Geometry check sheet. Reference: the model listing, model coordinates, mm. A direction names the side the tool comes from. Round coordinates to 2 decimals unless told otherwise and drop trailing zeros. Loops run counter-clockwise (first coordinate to the right, second up) from the corner with the lowest first, then second, coordinate; pieces in that order, holes last.
```python
from build123d import *

# Parameters (mm, degrees)
BOSS_EXTRUDE1_DEPTH      = 125
BOSS_EXTRUDE1_DEPTH_BACK = 75
SKETCH1_R                = 10
BOSS_EXTRUDE2_START      = 15
BOSS_EXTRUDE2_DEPTH      = 7.5
BODY_MOVE_COPY4_ANGLE    = 90
CUT_EXTRUDE1_START       = 10
CUT_EXTRUDE1_DEPTH       = 4
CUT_EXTRUDE1_DRAFT       = -5


with BuildPart() as part:
    # Sketch1 → Boss-Extrude1 (new, two sides: drawn at the far end of the back side and taken through both)
    with BuildSketch(Plane(origin=(0, 0, 0), x_dir=(0, 0, -1), z_dir=(1, 0, 0)).offset(-BOSS_EXTRUDE1_DEPTH_BACK)):
        Circle(SKETCH1_R)
    extrude(amount=BOSS_EXTRUDE1_DEPTH + BOSS_EXTRUDE1_DEPTH_BACK)

    # Sketch2 → Boss-Extrude2 (add, symmetric)
    with BuildSketch(Plane(origin=(0, 0, 0), x_dir=(0, 0, -1), z_dir=(1, 0, 0)).offset(BOSS_EXTRUDE2_START)):
        with BuildLine():
            ThreePointArc((-4.950818385, 10.931120589), (-10.855235073, -5.115063196), (5.27814522, -10.776881879))
            ThreePointArc((5.27814522, -10.776881879), (10.675009162, -7.586625818), (15.507108825, -3.59229396))
            ThreePointArc((15.507108825, -3.59229396), (16.895326586, -1.149524968), (16.746983201, 1.656230392))
            ThreePointArc((16.746983201, 1.656230392), (7.939134659, 11.068540296), (-4.950818385, 10.931120589))
        make_face()
    boss_extrude2 = extrude(amount=BOSS_EXTRUDE2_DEPTH, both=True)

    # Mirror3: Boss-Extrude2 across plane
    add(boss_extrude2.mirror(Plane(origin=(0, 0, 0), x_dir=(0, 0, 1), z_dir=(1, 0, 0))))


with BuildPart() as body_2:
    # Split1: the piece on the far side of the plane
    add(part.part)
    split(bisect_by=Plane(origin=(0, 0, 0), x_dir=(0, 0, 1), z_dir=(1, 0, 0)), keep=Keep.BOTTOM)


with BuildPart() as part_1:
    add(part.part)

    # Split1
    split(bisect_by=Plane(origin=(0, 0, 0), x_dir=(0, 0, 1), z_dir=(1, 0, 0)), keep=Keep.TOP)


with BuildPart() as body_2_1:
    # Body-Move/Copy4: moved
    add(body_2.part.rotate(Axis((0, 0, 0), (-1, 0, 0)), BODY_MOVE_COPY4_ANGLE))

    # Combine1: union part
    add(part_1.part)


with BuildPart() as cut_extrude1_tool:
    # Sketch5 → Cut-Extrude1 (with draft: the straight prism first)
    with BuildSketch(Plane(origin=(0, 0, 0), x_dir=(1, 0, 0), z_dir=(0, 1, 0)).offset(CUT_EXTRUDE1_START)):
        with BuildLine():
            ThreePointArc((97, 4), (93, 0), (97, -4))
            Line((97, -4), (117, -4))
            ThreePointArc((117, -4), (121, 0), (117, 4))
            Line((117, 4), (97, 4))
        make_face()
    extrude(amount=-CUT_EXTRUDE1_DEPTH)
    # Cut-Extrude1: the draft: its side faces are tilted about the plane it starts from
    cut_extrude1_sides = [cut_extrude1_tool.faces().sort_by_distance(p)[0] for p in [
        (121, 8, 0),
        (107, 8, -4),
        (93, 8, 0),
        (107, 8, 4),
    ]]
    draft(cut_extrude1_sides, Plane(origin=(0, 0, 0), x_dir=(1, 0, 0), z_dir=(0, 1, 0)).offset(CUT_EXTRUDE1_START), CUT_EXTRUDE1_DRAFT)


with BuildPart() as body_2_2:
    add(body_2_1.part)

    # Cut-Extrude1: cut by cut_extrude1_tool
    add(cut_extrude1_tool.part, mode=Mode.SUBTRACT)


solid = body_2_2.part
```
1) Scan lines: line 1 along X through (y, z) = (3.75, -10); line 2 along Z through (x, y) = (53, -0.75); line 3 along X through (y, z) = (6.5, -2). Record each from-to range of solid material in increasing order.
Report:
line 1: x = -22.5 to -7.5, 7.5 to 22.5
line 2: z = -9.97 to 9.97
line 3: x = -75 to 93.89, 120.11 to 125
2) Gauge pin test, flat ends, axial feed: pin 1 (8 mm diameter, centred on x = 112.5, z = 0.5, fed in from +Y); pin 2 (8 mm diameter, centred on x = -3, z = -2.5, fed in from +Y); pin 3 (8 mm diameter, centred on x = 67.5, y = -11.5, fed in from +Z). Record the tip position at first contact, or that the pin passes through.
Report:
pin 1: stops at y = 9.2
pin 2: stops at y = 10
pin 3: stops at z = 6.61
3) Sectioned sample at B-B, the plane x = -60.5. Record the cut outline in (y, z), then the cut area to 3 significant figures.
Report:
outline: circle Ø20 at (0, 0)
area: 314 mm2
4) Access from +Z, -Z, +X, -X, +Y, -Y to the whole of each face (thin tool, end or side, straight path). Record for faces 4 (the face through (22.5, 2, -10)), 5 (the face through (15.1, -7.64, -10.6)), 6 (the face through (120.788, 7.584, 0.083)), 7 (the face through (-22.5, -10, -2)), 8 (the face through (7.5, 2, -10)).
Report:
face 4: +X
face 5: -Z, +X, -Y
face 6: +Y
face 7: -X
face 8: none
5) Mould release check, pull along Z, two halves, no side actions. Record for faces 1 (the face through (-15.105, 10.966, 4.873)), 2 (the face through (107, 6, 0)), 3 (the face through (-15.1, -8.1, -11)): +Z half, -Z half, draft (parallel to the pull), parting line (faces both ways), or undercut.
Report:
face 1: parting line
face 2: undercut
face 3: -Z half
6) Sectioned sample at A-A, the plane x = -15. Record the cut outline in (y, z), then the cut area to 3 significant figures.
Report:
outline: (-16.75, -1.66) arc R16 ccw to (4.95, -10.93) arc R12 ccw (long way) to (-5.28, 10.78) arc R40 ccw to (-15.51, 3.59) arc R5 ccw to start
area: 533 mm2
